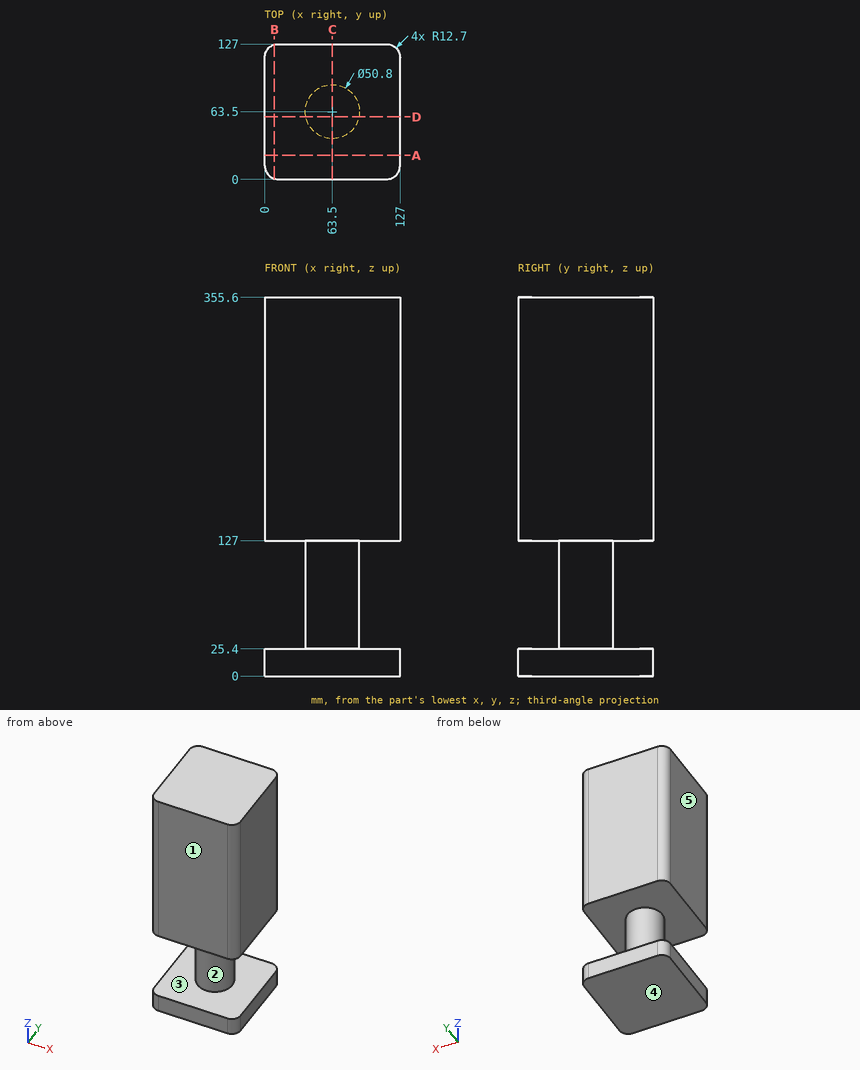
Could you check a few things on this drawing? It's one solid part, dimensions in mm from its lowest x, y, z. A direction names the side the tool comes from. Give positions to 0.01 mm unless a question says otherwise; leave off trailing zeros. Loops run counter-clockwise (first coordinate to the right, second up) from the corner with the lowest first, then second, coordinate; pieces in that order, holes last. Notation, with made-up numbers: M -27,-23.5 L -14,-23.5 A17 cw -14,-0.5 Z; hole C 5.5,27 d8. An arc over 180 degrees is marked long. One line per question, with ' | ' between items. Start each with the question number.
Q1. For pin 1 Ø3 at (y, z) = (48.5, 86.5) entering from -X; pin 2 Ø4 at (x, z) = (78, 65.5) entering from +Y, each with a flat end and sliding along its axis, tell me the tip position at first contact or that it passes through.
Q2. If we mould it in two halves opening along Z, with no side actions, what happens to the marked faces 3, 4 and 5? For each: +Z half, -Z half, draft (parallel to the pull), parting line (faces both ways), or undercut.
Q3. If we section it at D-D (y = 58.5): Please give me the cut outline in (x, z), plus the area to 3 significant figures.
Q4. If we section it at C-C (x = 63.5): Please give me the cut outline in (y, z), plus the area to 3 significant figures.
Q5. If we section it at B-B (x = 9): Please give me the cut outline in (y, z).
Q6. If I drill on line 1 (Z direction, x = 109.5, y = 48); line 2 (X direction, y = 7.5, z = 326), over which ranges is the centre line in solid material (lowest first)? Write a range as from..to.
Q7. If we section it at A-A (y = 22.5): Please give me the cut outline in (x, z).
Q8. For the marked faces 1 and 2, which set-ups out of +Z, -Z, +X, -X, +Y, -Y let a thin tool reach every point of the face, with its end or its side?
Computed:
1) pin 1: stops at x = 41.98 | pin 2: stops at y = 85.61
2) face 3: undercut | face 4: -Z half | face 5: draft
3) outline: M 0,0 L 127,0 L 127,25.4 L 88.4,25.4 L 88.4,127 L 127,127 L 127,355.6 L 0,355.6 L 0,127 L 38.6,127 L 38.6,25.4 L 0,25.4 Z | area: 37,300 mm²
4) outline: M 0,0 L 127,0 L 127,25.4 L 88.9,25.4 L 88.9,127 L 127,127 L 127,355.6 L 0,355.6 L 0,127 L 38.1,127 L 38.1,25.4 L 0,25.4 Z | area: 37,400 mm²
5) outline: M 0.55,0 L 126.45,0 L 126.45,25.4 L 0.55,25.4 Z; M 0.55,127 L 126.45,127 L 126.45,355.6 L 0.55,355.6 Z
6) line 1: z = 0..25.4, 127..355.6 | line 2: x = 1.11..125.89
7) outline: M 0,0 L 127,0 L 127,25.4 L 0,25.4 Z; M 0,127 L 127,127 L 127,355.6 L 0,355.6 Z
8) face 1: +Z, -Z, +X, -X, -Y | face 2: none
